```python
from build123d import *

# Parameters (mm, degrees)
SKETCH1_W                    = 189.8572
SKETCH1_H                    = 175.514
BASE_FLANGE1_DEPTH           = 2.3622
EDGE_FLANGE4_STRIP_W         = 11.0744
EDGE_FLANGE4_STRIP_H         = 2.3622
EDGE_FLANGE4_STRIP_CUT_DEPTH = 189.8572
EDGE_FLANGE4_DEPTH           = 189.8572
CUT_EXTRUDE1_DEPTH           = 145.352665205
CUT_EXTRUDE5_REACH           = 151.669
SKETCH41_R                   = 2.4765
CUT_EXTRUDE6_REACH           = 138.891
SKETCH42_R                   = 2.413


# Sheet-metal steps are written as plain solids
with BuildPart() as part:
    # Sketch1 → Base-Flange1 (new body)
    with BuildSketch(Plane(origin=(0, 0, 0), x_dir=(1, 0, 0), z_dir=(0, 1, 0))):
        with Locations((12.6128, 7.08)):
            Rectangle(SKETCH1_W, SKETCH1_H)
    extrude(amount=-BASE_FLANGE1_DEPTH)

    # Edge-Flange4 strip (across the edge) → Edge-Flange4 strip cut (cut)
    with BuildSketch(Plane(origin=(107.5414, -2.3622, 80.677), x_dir=(0, 0, -1), z_dir=(-1, 0, 0))):
        with Locations((-4.7244, -1.1811)):
            Rectangle(EDGE_FLANGE4_STRIP_W, EDGE_FLANGE4_STRIP_H)
    extrude(amount=EDGE_FLANGE4_STRIP_CUT_DEPTH, mode=Mode.SUBTRACT)

    # Edge-Flange4 section (across the edge) → Edge-Flange4 (add)
    with BuildSketch(Plane(origin=(107.5414, -2.3622, 80.677), x_dir=(0, 0, -1), z_dir=(-1, 0, 0))):
        with BuildLine():
            Line((-2.3622, 0.8128), (-2.3622, 16.6878))
            Line((-2.3622, 16.6878), (0, 16.6878))
            Line((0, 16.6878), (0, 0.8128))
            ThreePointArc((0, 0.8128), (0.238063608, 0.238063608), (0.8128, 0))
            Line((0.8128, 0), (0.8128, -2.3622))
            ThreePointArc((0.8128, -2.3622), (-1.43226403, -1.43226403), (-2.3622, 0.8128))
        make_face()
    extrude(amount=EDGE_FLANGE4_DEPTH)

    # Sketch36 → Cut-Extrude1 (cut, through all)
    with BuildSketch(Plane.XZ.offset(2.3622)):
        Polygon((20.98856689, -21.6596), (-82.3158, -21.6596), (-82.3158, -94.837), (107.5414, -94.837), (107.5414, 50.96685034), align=None)
    extrude(amount=-CUT_EXTRUDE1_DEPTH, mode=Mode.SUBTRACT)

    # Sketch41 → Cut-Extrude5 (cut, up to next)
    with BuildSketch(Plane(origin=(0, 0, 80.677), x_dir=(-1, 0, 0), z_dir=(0, 0, -1)), mode=Mode.PRIVATE) as cut_extrude5_sk1:
        with Locations(Location((-88.8128, -11.1125, 0), (0, 0, 90))):
            Circle(SKETCH41_R)
    cut_extrude5_tool1 = extrude(cut_extrude5_sk1.sketch, amount=-CUT_EXTRUDE5_REACH, mode=Mode.PRIVATE) & part.part
    # Sketch41 → Cut-Extrude5 (cut, up to next)
    with BuildSketch(Plane(origin=(0, 0, 80.677), x_dir=(-1, 0, 0), z_dir=(0, 0, -1)), mode=Mode.PRIVATE) as cut_extrude5_sk2:
        with Locations(Location((-63.4128, -11.1125, 0), (0, 0, 90))):
            Circle(SKETCH41_R)
    cut_extrude5_tool2 = extrude(cut_extrude5_sk2.sketch, amount=-CUT_EXTRUDE5_REACH, mode=Mode.PRIVATE) & part.part
    # Sketch41 → Cut-Extrude5 (cut, up to next)
    with BuildSketch(Plane(origin=(0, 0, 80.677), x_dir=(-1, 0, 0), z_dir=(0, 0, -1)), mode=Mode.PRIVATE) as cut_extrude5_sk3:
        with Locations(Location((-38.0128, -11.1125, 0), (0, 0, 90))):
            Circle(SKETCH41_R)
    cut_extrude5_tool3 = extrude(cut_extrude5_sk3.sketch, amount=-CUT_EXTRUDE5_REACH, mode=Mode.PRIVATE) & part.part
    # Sketch41 → Cut-Extrude5 (cut, up to next)
    with BuildSketch(Plane(origin=(0, 0, 80.677), x_dir=(-1, 0, 0), z_dir=(0, 0, -1)), mode=Mode.PRIVATE) as cut_extrude5_sk4:
        with Locations(Location((-12.6128, -11.1125, 0), (0, 0, 90))):
            Circle(SKETCH41_R)
    cut_extrude5_tool4 = extrude(cut_extrude5_sk4.sketch, amount=-CUT_EXTRUDE5_REACH, mode=Mode.PRIVATE) & part.part
    # Sketch41 → Cut-Extrude5 (cut, up to next)
    with BuildSketch(Plane(origin=(0, 0, 80.677), x_dir=(-1, 0, 0), z_dir=(0, 0, -1)), mode=Mode.PRIVATE) as cut_extrude5_sk5:
        with Locations(Location((12.7872, -11.1125, 0), (0, 0, 90))):
            Circle(SKETCH41_R)
    cut_extrude5_tool5 = extrude(cut_extrude5_sk5.sketch, amount=-CUT_EXTRUDE5_REACH, mode=Mode.PRIVATE) & part.part
    # Sketch41 → Cut-Extrude5 (cut, up to next)
    with BuildSketch(Plane(origin=(0, 0, 80.677), x_dir=(-1, 0, 0), z_dir=(0, 0, -1)), mode=Mode.PRIVATE) as cut_extrude5_sk6:
        with Locations(Location((38.1872, -11.1125, 0), (0, 0, 90))):
            Circle(SKETCH41_R)
    cut_extrude5_tool6 = extrude(cut_extrude5_sk6.sketch, amount=-CUT_EXTRUDE5_REACH, mode=Mode.PRIVATE) & part.part
    # Sketch41 → Cut-Extrude5 (cut, up to next)
    with BuildSketch(Plane(origin=(0, 0, 80.677), x_dir=(-1, 0, 0), z_dir=(0, 0, -1)), mode=Mode.PRIVATE) as cut_extrude5_sk7:
        with Locations(Location((63.5872, -11.1125, 0), (0, 0, 90))):
            Circle(SKETCH41_R)
    cut_extrude5_tool7 = extrude(cut_extrude5_sk7.sketch, amount=-CUT_EXTRUDE5_REACH, mode=Mode.PRIVATE) & part.part
    add(cut_extrude5_tool1.solids().sort_by_distance((88.8128, -11.1125, 80.677))[0], mode=Mode.SUBTRACT)
    add(cut_extrude5_tool2.solids().sort_by_distance((63.4128, -11.1125, 80.677))[0], mode=Mode.SUBTRACT)
    add(cut_extrude5_tool3.solids().sort_by_distance((38.0128, -11.1125, 80.677))[0], mode=Mode.SUBTRACT)
    add(cut_extrude5_tool4.solids().sort_by_distance((12.6128, -11.1125, 80.677))[0], mode=Mode.SUBTRACT)
    add(cut_extrude5_tool5.solids().sort_by_distance((-12.7872, -11.1125, 80.677))[0], mode=Mode.SUBTRACT)
    add(cut_extrude5_tool6.solids().sort_by_distance((-38.1872, -11.1125, 80.677))[0], mode=Mode.SUBTRACT)
    add(cut_extrude5_tool7.solids().sort_by_distance((-63.5872, -11.1125, 80.677))[0], mode=Mode.SUBTRACT)

    # Sketch42 → Cut-Extrude6 (cut, up to next)
    with BuildSketch(Plane.XZ.offset(2.3622), mode=Mode.PRIVATE) as cut_extrude6_sk1:
        with Locations(Location((-74.3402, -8.2596, 0), (0, 0, 270))):
            Circle(SKETCH42_R)
    cut_extrude6_tool1 = extrude(cut_extrude6_sk1.sketch, amount=-CUT_EXTRUDE6_REACH, mode=Mode.PRIVATE) & part.part
    # Sketch42 → Cut-Extrude6 (cut, up to next)
    with BuildSketch(Plane.XZ.offset(2.3622), mode=Mode.PRIVATE) as cut_extrude6_sk2:
        with Locations(Location((-74.3402, 17.1404, 0), (0, 0, 270))):
            Circle(SKETCH42_R)
    cut_extrude6_tool2 = extrude(cut_extrude6_sk2.sketch, amount=-CUT_EXTRUDE6_REACH, mode=Mode.PRIVATE) & part.part
    # Sketch42 → Cut-Extrude6 (cut, up to next)
    with BuildSketch(Plane.XZ.offset(2.3622), mode=Mode.PRIVATE) as cut_extrude6_sk3:
        with Locations(Location((-74.3402, 42.5404, 0), (0, 0, 270))):
            Circle(SKETCH42_R)
    cut_extrude6_tool3 = extrude(cut_extrude6_sk3.sketch, amount=-CUT_EXTRUDE6_REACH, mode=Mode.PRIVATE) & part.part
    # Sketch42 → Cut-Extrude6 (cut, up to next)
    with BuildSketch(Plane.XZ.offset(2.3622), mode=Mode.PRIVATE) as cut_extrude6_sk4:
        with Locations(Location((-74.3402, 67.9404, 0), (0, 0, 270))):
            Circle(SKETCH42_R)
    cut_extrude6_tool4 = extrude(cut_extrude6_sk4.sketch, amount=-CUT_EXTRUDE6_REACH, mode=Mode.PRIVATE) & part.part
    # Sketch42 → Cut-Extrude6 (cut, up to next)
    with BuildSketch(Plane.XZ.offset(2.3622), mode=Mode.PRIVATE) as cut_extrude6_sk5:
        with Locations(Location((99.5658, 59.3432, 0), (0, 0, 270))):
            Circle(SKETCH42_R)
    cut_extrude6_tool5 = extrude(cut_extrude6_sk5.sketch, amount=-CUT_EXTRUDE6_REACH, mode=Mode.PRIVATE) & part.part
    # Sketch42 → Cut-Extrude6 (cut, up to next)
    with BuildSketch(Plane.XZ.offset(2.3622), mode=Mode.PRIVATE) as cut_extrude6_sk6:
        with Locations(Location((99.5658, 72.0432, 0), (0, 0, 270))):
            Circle(SKETCH42_R)
    cut_extrude6_tool6 = extrude(cut_extrude6_sk6.sketch, amount=-CUT_EXTRUDE6_REACH, mode=Mode.PRIVATE) & part.part
    add(cut_extrude6_tool1.solids().sort_by_distance((-74.3402, -2.3622, -8.2596))[0], mode=Mode.SUBTRACT)
    add(cut_extrude6_tool2.solids().sort_by_distance((-74.3402, -2.3622, 17.1404))[0], mode=Mode.SUBTRACT)
    add(cut_extrude6_tool3.solids().sort_by_distance((-74.3402, -2.3622, 42.5404))[0], mode=Mode.SUBTRACT)
    add(cut_extrude6_tool4.solids().sort_by_distance((-74.3402, -2.3622, 67.9404))[0], mode=Mode.SUBTRACT)
    add(cut_extrude6_tool5.solids().sort_by_distance((99.5658, -2.3622, 59.3432))[0], mode=Mode.SUBTRACT)
    add(cut_extrude6_tool6.solids().sort_by_distance((99.5658, -2.3622, 72.0432))[0], mode=Mode.SUBTRACT)


solid = part.part
```
Could you check a few things on this model? Use its own coordinates, in mm. A direction names the side the tool comes from. Coordinates: 2 decimals unless noted, no trailing zeros. Loops run counter-clockwise (first coordinate to the right, second up) from the corner with the lowest first, then second, coordinate; pieces in that order, holes last.
1) Thinking about a two-plate mould opening in Z: for faces 1 (the face through (88.922, -13.587, 81.842)), 2 (the face through (-76.481, -1.198, 66.827)), 3 (the face through (14, -8, 80.677)), which applies, released by +Z, released by -Z, zero draft, split by the parting line, or undercut?
Reported:
face 1: zero draft
face 2: undercut
face 3: released by -Z
2) Which directions (+Z, -Z, +X, -X, +Y, -Y) give clear straight access to the entire face, cutting with the end or side of a thin tool? Please do faces 4 (the face through (-10, -2.362, 28)), 5 (the face through (-61.913, -12.938, 81.842)).
Reported:
face 4: -Z, +X, -X, -Y
face 5: +Z, -Z
3) Please list where these lines run through material, in increasing order: line 1 along Y through (x, z) = (34, 27.5); line 2 along Z through (x, y) = (49, -11); line 3 along X through (y, z) = (-1.5, -15).
Reported:
line 1: y = -2.36 to 0
line 2: z = 80.68 to 83.04
line 3: x = -82.32 to 28.93
4) Will these pins go through, and if not, where does the flat tip stop? pin 1 Ø6.5 at (x, y) = (38.01, -11.11) entering from +Z; pin 2 Ø2 at (x, y) = (-41, -13.5) entering from -Z; pin 3 Ø4.5 at (x, z) = (-74.34, 17.14) entering from +Y; pin 4 Ø4 at (x, z) = (41, 58) entering from -Y.
Reported:
pin 1: stops at z = 83.04
pin 2: stops at z = 80.68
pin 3: passes through
pin 4: stops at y = -2.36
5) Imagine slicing it at C-C (z = 17). List the corners of the cut face in (x, y) for me.
Reported:
outline: (-82.32, -2.36) - (-76.75, -2.36) - (-76.75, 0) - (-82.32, 0) - close; (-71.93, -2.36) - (67.06, -2.36) - (67.06, 0) - (-71.93, 0) - close
6) Imagine slicing it at B-B (x = 6). List the corners of the cut face in (y, z) for me (3 decimals), and give its area (3 significant figures).
Reported:
outline: (-19.05, 80.677) - (-3.175, 80.677) arc R0.813 cw to (-2.362, 79.864) - (-2.362, -21.66) - (0, -21.66) - (0, 79.864) arc R3.175 ccw to (-3.175, 83.039) - (-19.05, 83.039) - close
area: 285 mm2
7) Imagine slicing it at A-A (z = -8). List the corners of the cut face in (x, y) for me, and give its area (3 significant figures).
Reported:
outline: (-82.32, -2.36) - (-76.74, -2.36) - (-76.74, 0) - (-82.32, 0) - close; (-71.94, -2.36) - (37.27, -2.36) - (37.27, 0) - (-71.94, 0) - close
area: 271 mm2
8) Imagine slicing it at D-D (x = 32). List the corners of the cut face in (y, z) for me (3 decimals), and give its area (3 significant figures).
Reported:
outline: (-19.05, 80.677) - (-3.175, 80.677) arc R0.813 cw to (-2.362, 79.864) - (-2.362, -12.42) - (0, -12.42) - (0, 79.864) arc R3.175 ccw to (-3.175, 83.039) - (-19.05, 83.039) - close
area: 263 mm2
